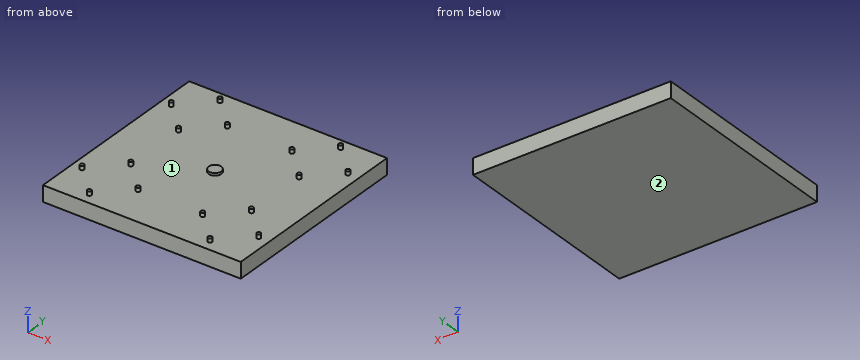
from build123d import *

# Parameters (mm, degrees)
F0_W            = 1995
F0_H            = 1995
F1_DEPTH        = 160
F2_R            = 20
F3_DEPTH        = 40
F3_COPIES_COUNT = 4
F4_R            = 63.875346373
F5_DEPTH        = 25


# Not quite as in the source:
# - a pattern or mirror of a feature is missing from the dataset's text; its kind, count and spacing are read off the source's solid


with BuildPart() as f1:
    # F0 (on Top) → F1 (new body)
    with BuildSketch(Plane.XY):
        Rectangle(F0_W, F0_H)
    extrude(amount=F1_DEPTH)

    # F2 (on face) → F3 (join)
    with BuildSketch(Plane.XY.offset(160)):
        with Locations((-608.5912703474, 891.433982822)):
            Circle(F2_R)
        with Locations((-325.7485578728, 608.5912703474)):
            Circle(F2_R)
        with Locations((-608.5912703474, 325.7485578728)):
            Circle(F2_R)
        with Locations((-891.433982822, 608.5912703474)):
            Circle(F2_R)
    f3 = extrude(amount=F3_DEPTH)

    # F3_copies: F3 ×4 about axis
    f3_copies_axis = Axis((0, 0, 0), (0, 0, 1))
    for i in range(1, F3_COPIES_COUNT):
        add(f3.rotate(f3_copies_axis, i * 360 / F3_COPIES_COUNT))

    # F4 (on face) → F5 (join)
    with BuildSketch(Plane.XY.offset(160)):
        Circle(F4_R)
    extrude(amount=F5_DEPTH)


solid = f1.part
Source: CAD feature listing. Evaluate the final solid. Frame: model axes, mm. Face numbers are marked on the shaded views. A direction names the side the tool comes from. Round coordinates to 2 decimals unless told otherwise and drop trailing zeros. Order: outer loops, then holes, each group sorted by start corner. A loop starts at its lowest first (then second) coordinate and runs counter-clockwise, first axis right, second up. Notation, with made-up numbers: (0, 83) -> (51, 83) arc R14 cw to (51, 96) -> close; hole circle Ø2 at (82, 48.25). An arc over 180 degrees is marked (long way). Answer as CSV lines item,"result".
Item 1: Line query: L1, parallel to Z at x = -156, y = -732; L2, parallel to Y at x = 624, z = 184. Output: solid intervals per line, ascending.
A:
L1,"0 to 160"
L2,"-904.18 to -878.68, -338.5 to -313, 313 to 338.5, 878.68 to 904.18"
Item 2: Reachability of the marked faces 1 and 2 from +Z, -Z, +X, -X, +Y, -Y: full face, straight path, thin tool, end or side. Return the list, or none.
A:
face 1,"+Z"
face 2,"-Z, +X, -X, +Y, -Y"
Item 3: Pin query (flat end, axial travel): pin 1 Ø6 at (x, z) = (425.5, 165.5) entering from +Y; pin 2 Ø12 at (x, y) = (-768.5, -744) entering from +Z. Return the tip coordinate at first contact, or that it passes through.
A:
pin 1,"through"
pin 2,"z = 160"
Item 4: Section C-C, the plane y = 542. Return loops of the section in (x, z).
A:
outline,"(-997.5, 0) -> (997.5, 0) -> (997.5, 160) -> (-997.5, 160) -> close"
Item 5: Section A-A, the plane y = 0. Return loops of the section in (x, z).
A:
outline,"(-997.5, 0) -> (997.5, 0) -> (997.5, 160) -> (63.88, 160) -> (63.88, 185) -> (-63.88, 185) -> (-63.88, 160) -> (-997.5, 160) -> close"
